Model file for the job. Use its own axes, mm. A direction names the side the tool comes from. Round coordinates to 2 decimals unless told otherwise and drop trailing zeros. Loops run counter-clockwise (first coordinate to the right, second up) from the corner with the lowest first, then second, coordinate; pieces in that order, holes last. Notation, with made-up numbers: (14.5, -4.5) -> (72.5, -4.5) arc R30 cw to (72.5, 26.5) -> close; hole circle Ø4 at (33.25, 20). An arc over 180 degrees is marked (long way). Use a Markdown table: item, result.
from build123d import *

# Parameters (mm, degrees)
F1_DEPTH = 7.8
F3_DEPTH = 5


with BuildPart() as f1:
    # F0 (on Top) → F1 (new body)
    with BuildSketch(Plane.XY):
        with BuildLine():
            Line((39.1, -70.15), (39.1, 70.15))
            ThreePointArc((39.1, 70.15), (37.342641, 74.392641), (33.1, 76.15))
            Line((33.1, 76.15), (-33.1, 76.15))
            ThreePointArc((-33.1, 76.15), (-37.342641, 74.392641), (-39.1, 70.15))
            Line((-39.1, 70.15), (-39.1, -70.15))
            ThreePointArc((-39.1, -70.15), (-37.342641, -74.392641), (-33.1, -76.15))
            Line((-33.1, -76.15), (33.1, -76.15))
            ThreePointArc((33.1, -76.15), (37.342641, -74.392641), (39.1, -70.15))
        make_face()
        with BuildLine():
            Line((-33.1, 73.15), (33.1, 73.15))
            ThreePointArc((33.1, 73.15), (35.22132, 72.27132), (36.1, 70.15))
            Line((36.1, 70.15), (36.1, -70.15))
            ThreePointArc((36.1, -70.15), (35.22132, -72.27132), (33.1, -73.15))
            Line((33.1, -73.15), (-33.1, -73.15))
            ThreePointArc((-33.1, -73.15), (-35.22132, -72.27132), (-36.1, -70.15))
            Line((-36.1, -70.15), (-36.1, 70.15))
            ThreePointArc((-36.1, 70.15), (-35.22132, 72.27132), (-33.1, 73.15))
        make_face(mode=Mode.SUBTRACT)
    extrude(amount=F1_DEPTH)

    # F2 (on face) → F3 (join)
    with BuildSketch(Plane(origin=(0, 0, 0), x_dir=(1, 0, 0), z_dir=(0, 0, -1))):
        with BuildLine():
            Line((-4.203966, 31.27091), (-31.168408, 73.15))
            Line((-31.168408, 73.15), (-33.1, 73.15))
            ThreePointArc((-33.1, 73.15), (-35.22132, 72.27132), (-36.1, 70.15))
            Line((-36.1, 70.15), (-36.1, 59.508006))
            Line((-36.1, 59.508006), (-19.707009, 1.356636))
            ThreePointArc((-19.707009, 1.356636), (-19.519445, 0), (-19.707009, -1.356636))
            Line((-19.707009, -1.356636), (-36.1, -59.508006))
            Line((-36.1, -59.508006), (-36.1, -70.15))
            ThreePointArc((-36.1, -70.15), (-35.22132, -72.27132), (-33.1, -73.15))
            Line((-33.1, -73.15), (-31.168408, -73.15))
            Line((-31.168408, -73.15), (-4.203966, -31.27091))
            ThreePointArc((-4.203966, -31.27091), (0, -28.977692), (4.203966, -31.27091))
            Line((4.203966, -31.27091), (31.168408, -73.15))
            Line((31.168408, -73.15), (33.1, -73.15))
            ThreePointArc((33.1, -73.15), (35.22132, -72.27132), (36.1, -70.15))
            Line((36.1, -70.15), (36.1, -59.508006))
            Line((36.1, -59.508006), (19.707009, -1.356636))
            ThreePointArc((19.707009, -1.356636), (19.519445, 0), (19.707009, 1.356636))
            Line((19.707009, 1.356636), (36.1, 59.508006))
            Line((36.1, 59.508006), (36.1, 70.15))
            ThreePointArc((36.1, 70.15), (35.22132, 72.27132), (33.1, 73.15))
            Line((33.1, 73.15), (31.168408, 73.15))
            Line((31.168408, 73.15), (4.203966, 31.27091))
            ThreePointArc((4.203966, 31.27091), (0, 28.977692), (-4.203966, 31.27091))
        make_face()
        with BuildLine():
            Line((-31.168408, 73.15), (-33.1, 76.15))
            ThreePointArc((-33.1, 76.15), (-37.342641, 74.392641), (-39.1, 70.15))
            Line((-39.1, 70.15), (-36.1, 59.508006))
            Line((-36.1, 59.508006), (-36.1, 70.15))
            ThreePointArc((-36.1, 70.15), (-35.22132, 72.27132), (-33.1, 73.15))
            Line((-33.1, 73.15), (-31.168408, 73.15))
        make_face()
        with BuildLine():
            ThreePointArc((39.1, 70.15), (37.342641, 74.392641), (33.1, 76.15))
            Line((33.1, 76.15), (31.168408, 73.15))
            Line((31.168408, 73.15), (33.1, 73.15))
            ThreePointArc((33.1, 73.15), (35.22132, 72.27132), (36.1, 70.15))
            Line((36.1, 70.15), (36.1, 59.508006))
            Line((36.1, 59.508006), (39.1, 70.15))
        make_face()
        with BuildLine():
            ThreePointArc((33.1, -76.15), (37.342641, -74.392641), (39.1, -70.15))
            Line((39.1, -70.15), (36.1, -59.508006))
            Line((36.1, -59.508006), (36.1, -70.15))
            ThreePointArc((36.1, -70.15), (35.22132, -72.27132), (33.1, -73.15))
            Line((33.1, -73.15), (31.168408, -73.15))
            Line((31.168408, -73.15), (33.1, -76.15))
        make_face()
        with BuildLine():
            Line((-36.1, -59.508006), (-39.1, -70.15))
            ThreePointArc((-39.1, -70.15), (-37.342641, -74.392641), (-33.1, -76.15))
            Line((-33.1, -76.15), (-31.168408, -73.15))
            Line((-31.168408, -73.15), (-33.1, -73.15))
            ThreePointArc((-33.1, -73.15), (-35.22132, -72.27132), (-36.1, -70.15))
            Line((-36.1, -70.15), (-36.1, -59.508006))
        make_face()
    extrude(amount=F3_DEPTH)


solid = f1.part
Q1. Band-saw the part on D-D, the plane y = -10.5. Give the cut face in (x, z).
Results list:
| item | result |
|---|---|
| outline | (-39.1, 0) -> (-36.1, 0) -> (-36.1, 7.8) -> (-39.1, 7.8) -> close; (-22.28, -5) -> (22.28, -5) -> (22.28, 0) -> (-22.28, 0) -> close; (36.1, 0) -> (39.1, 0) -> (39.1, 7.8) -> (36.1, 7.8) -> close |
Q2. Band-saw the part on C-C, the plane x = 12.5. Give the cut face in (y, z), plus the area to 3 significant figures.
Results list:
| item | result |
|---|---|
| outline | (-76.15, 0) -> (-73.15, 0) -> (-73.15, 7.8) -> (-76.15, 7.8) -> close; (-44.16, -5) -> (44.16, -5) -> (44.16, 0) -> (-44.16, 0) -> close; (73.15, 0) -> (76.15, 0) -> (76.15, 7.8) -> (73.15, 7.8) -> close |
| area | 488 mm² |
Q3. Band-saw the part on A-A, the plane z = 2. Give the cut face in (x, y).
Results list:
| item | result |
|---|---|
| outline | (-39.1, -70.15) arc R6 ccw to (-33.1, -76.15) -> (33.1, -76.15) arc R6 ccw to (39.1, -70.15) -> (39.1, 70.15) arc R6 ccw to (33.1, 76.15) -> (-33.1, 76.15) arc R6 ccw to (-39.1, 70.15) -> close; hole (-36.1, -70.15) arc R3 ccw to (-33.1, -73.15) -> (33.1, -73.15) arc R3 ccw to (36.1, -70.15) -> (36.1, 70.15) arc R3 ccw to (33.1, 73.15) -> (-33.1, 73.15) arc R3 ccw to (-36.1, 70.15) -> close |
Q4. Tool access for faces 1 (the face through (-36.1, -1, 4)), 2 (the face through (0, 75, 0)), 3 (the face through (-38, 23, 7.8)): list every direction of +Z, -Z, +X, -X, +Y, -Y with a clear straight run to the whole face (end or side of a thin tool).
Results list:
| item | result |
|---|---|
| face 1 | +Z |
| face 2 | -Z, +Y |
| face 3 | +Z, +X, -X, +Y, -Y |
Q5. Flat gauge pins, fed straight in: pin 1 (0.9 mm diameter, centred on x = -10.5, y = -74.5, fed in from -Z); pin 2 (2 mm diameter, centred on x = -24.5, z = -2.5, fed in from +Y); pin 3 (4 mm diameter, centred on x = 6.5, z = -2.5, fed in from -Y). Where does each tip first touch, or does it go through?
Results list:
| item | result |
|---|---|
| pin 1 | stops at z = 0 |
| pin 2 | stops at y = 64.35 |
| pin 3 | stops at y = -37.94 |
Q6. Pull direction X, two halves, no side cores. Call faces 4 (the face through (19.52, 0.02, -2.46)), 5 (the face through (0, -73.15, 4)), 6 (the face through (-39.1, 1, 4)): released by +X, released by -X, zero draft, split by the parting line, or undercut.
Results list:
| item | result |
|---|---|
| face 4 | released by +X |
| face 5 | undercut |
| face 6 | released by -X |
Q7. Drill centre lines: L1, parallel to Y at x = -1, z = 3.5; L2, parallel to Y at x = -33.5, z = 1.25; L3, parallel to X at y = 69, z = 5. Where is each one in solid material? Low to high. Write a range as from..to.
Results list:
| item | result |
|---|---|
| L1 | y = -76.15..-73.15, 73.15..76.15 |
| L2 | y = -76.14..-73.12, 73.12..76.14 |
| L3 | x = -39.1..-36.1, 36.1..39.1 |
Q8. Band-saw the part on B-B, the plane y = 41.5. Give the cut face in (x, z), plus the area to 3 significant figures.
Results list:
| item | result |
|---|---|
| outline | (-39.1, 0) -> (-36.1, 0) -> (-36.1, 7.8) -> (-39.1, 7.8) -> close; (-31.02, -5) -> (-10.79, -5) -> (-10.79, 0) -> (-31.02, 0) -> close; (10.79, -5) -> (31.02, -5) -> (31.02, 0) -> (10.79, 0) -> close; (36.1, 0) -> (39.1, 0) -> (39.1, 7.8) -> (36.1, 7.8) -> close |
| area | 249 mm² |
